Geometry: final body of the model. Coordinates: model frame, mm. Give positions to 0.01 mm unless a question says otherwise; leave off trailing zeros. Use a Markdown table: item, result. Add a question column.
1) Line query: line 1 (Z direction, x = 88.9, y = 11.25); line 2 (X direction, y = 8.75, z = -203.2). Output: solid intervals per line, ascending.
2) Pin query (flat end, axial travel): pin 1 (5.5 mm diameter, centred on x = 88.9, z = -203.2, fed in from +Y). Return the tip coordinate at first contact, or that it passes through.
3) Draft query along X for faces 1 (the flat face through (50, 10, 0)), 2 (the cylindrical face through (86.04, 9.86, -13.6)), 3 (the cylindrical face through (97.98, 10.14, -212.08)). Return one class per face: +X half, -X half, draft (parallel to the pull), parting line (faces both ways), or undercut.
```python
from build123d import *

# Parameters (mm, degrees)
SKETCH1_W           = 101.6
SKETCH1_H           = 215.9
BOSS_EXTRUDE2_DEPTH = 20
FILLET1_R           = 12.7
SKETCH5_R           = 3
CUT_EXTRUDE1_DEPTH  = 21


with BuildPart() as part:
    # Sketch1 → Boss-Extrude2 (new body)
    with BuildSketch(Plane(origin=(0, 0, 0), x_dir=(1, 0, 0), z_dir=(0, 1, 0))):
        with Locations((50.8, 107.95)):
            Rectangle(SKETCH1_W, SKETCH1_H)
    extrude(amount=BOSS_EXTRUDE2_DEPTH)

    # Fillet1
    fillet1_edges = [part.edges().sort_by_distance(p)[0] for p in [
        (0, 10, -215.9),
        (101.6, 10, -215.9),
        (101.6, 10, 0),
        (0, 10, 0),
    ]]
    fillet(fillet1_edges, radius=FILLET1_R)

    # Sketch5 → Cut-Extrude1 (cut, through all)
    with BuildSketch(Plane(origin=(0, 0, 0), x_dir=(-1, 0, 0), z_dir=(0, -1, 0))):
        with Locations((-88.9, 203.2)):
            Circle(SKETCH5_R)
        with Locations((-12.7, 203.2)):
            Circle(SKETCH5_R)
        with Locations((-88.9, 12.7)):
            Circle(SKETCH5_R)
        with Locations((-12.7, 12.7)):
            Circle(SKETCH5_R)
    extrude(amount=-CUT_EXTRUDE1_DEPTH, mode=Mode.SUBTRACT)


solid = part.part
```
Found:
| question | item | result |
|---|---|---|
| 1 | line 1 | -215.9 to -206.2, -200.2 to -15.7, -9.7 to 0 |
| 1 | line 2 | 0 to 9.7, 15.7 to 85.9, 91.9 to 101.6 |
| 2 | pin 1 | through |
| 3 | face 1 | draft |
| 3 | face 2 | undercut |
| 3 | face 3 | +X half |
